```python
from build123d import *

# Parameters (mm, degrees)
SKETCH1_R           = 1.5
BOSS_EXTRUDE1_DEPTH = 0.5
SKETCH2_W           = 16.871696
SKETCH2_H           = 4.360926
SKETCH2_W_2         = 4.86899
SKETCH2_H_2         = 12.600052
CUT_EXTRUDE2_DEPTH  = 37.229212531
FILLET1_R           = 1
SKETCH3_R           = 1
SKETCH3_W           = 1.5
SKETCH3_H           = 4
SKETCH3_R_2         = 1.5
BOSS_EXTRUDE2_DEPTH = 2.05
FILLET2_R           = 1
FILLET4_R           = 0.75


# Some blends are built 0.0001 mm under size
with BuildPart() as part:
    # Sketch1 → Boss-Extrude1 (new body)
    with BuildSketch(Plane.XZ.offset(3.35)):
        with BuildLine():
            Line((-30.468062, -16.001619), (30.468062, -16.001619))
            ThreePointArc((30.468062, -16.001619), (31.904902979, -15.406459979), (32.500062, -13.969619))
            Line((32.500062, -13.969619), (32.500062, 13.969619))
            ThreePointArc((32.500062, 13.969619), (31.904902979, 15.406459979), (30.468062, 16.001619))
            Line((30.468062, 16.001619), (-30.468062, 16.001619))
            ThreePointArc((-30.468062, 16.001619), (-31.904902979, 15.406459979), (-32.500062, 13.969619))
            Line((-32.500062, 13.969619), (-32.500062, -13.969619))
            ThreePointArc((-32.500062, -13.969619), (-31.904902979, -15.406459979), (-30.468062, -16.001619))
        make_face()
        with Locations(Location((28.999942, -11.463655, 0), (0, 0, 270))):
            Circle(SKETCH1_R, mode=Mode.SUBTRACT)
        with Locations(Location((28.999942, 11.536299, 0), (0, 0, 270))):
            Circle(SKETCH1_R, mode=Mode.SUBTRACT)
        with Locations(Location((-29.000196, -11.463655, 0), (0, 0, 270))):
            Circle(SKETCH1_R, mode=Mode.SUBTRACT)
        with Locations(Location((-29.000196, 11.536299, 0), (0, 0, 270))):
            Circle(SKETCH1_R, mode=Mode.SUBTRACT)
    extrude(amount=-BOSS_EXTRUDE1_DEPTH)

    # Sketch2 → Cut-Extrude2 (cut, through all)
    with BuildSketch(Plane.XZ.offset(3.35)):
        with Locations((-4.81203, 13.821156)):
            Rectangle(SKETCH2_W, SKETCH2_H)
        Polygon((-20.66863, -8.001619), (10.02857, -8.001619), (10.02857, -16.001619), (-25.94464, -16.001619), (-25.94464, -11.279987), (-20.66863, -11.279987), align=None)
        with Locations((30.065567, 1.825117)):
            Rectangle(SKETCH2_W_2, SKETCH2_H_2)
    extrude(amount=-CUT_EXTRUDE2_DEPTH, mode=Mode.SUBTRACT)

    # Fillet1
    fillet1_edges = [part.edges().sort_by_distance(p)[0] for p in [
        (-13.247878, -3.1, 16.001619),
        (3.623818, -3.1, 16.001619),
        (-20.66863, -3.1, -11.279987),
        (10.02857, -3.1, -16.001619),
        (-25.94464, -3.1, -16.001619),
        (32.500062, -3.1, 8.125143),
        (32.500062, -3.1, -4.474909),
    ]]
    fillet(fillet1_edges, radius=FILLET1_R)

    # Sketch3 → Boss-Extrude2 (add)
    # profile 1 of 9: a face of its own
    with BuildSketch(Plane.XZ.offset(3.35)):
        with Locations(Location((-12.947878, 8.140693, 0), (0, 0, 270))):
            Circle(SKETCH3_R)
    # profile 2 of 9: a face of its own
    with BuildSketch(Plane.XZ.offset(3.35)):
        with Locations(Location((-18.447878, 15.001619, 0), (0, 0, 90))):
            Circle(SKETCH3_R)
    # profile 3 of 9: a face of its own
    with BuildSketch(Plane.XZ.offset(3.35)):
        with Locations(Location((5.356479, 14.268958, 0), (0, 0, 270))):
            Circle(SKETCH3_R)
    # profile 4 of 9: a face of its own
    with BuildSketch(Plane.XZ.offset(3.35)):
        Polygon((-20.46863, -8.001619), (9.02857, -8.001619), (9.02857, -6.501619), (4.02857, -6.501619), (4.02857, 8.498381), (7.52857, 8.498381), (7.52857, 9.998381), (-0.47143, 9.998381), (-0.47143, 8.498381), (2.52857, 8.498381), (2.52857, -6.501619), (-20.46863, -6.501619), align=None)
    # profile 5 of 9: a face of its own
    with BuildSketch(Plane.XZ.offset(3.35)):
        with Locations((15.204059, 14.001619)):
            Rectangle(SKETCH3_W, SKETCH3_H)
    # profile 6 of 9: a face of its own
    with BuildSketch(Plane.XZ.offset(3.35)):
        with BuildLine():
            Line((-32.500062, -3.797223), (-32.500062, -13.969619))
            ThreePointArc((-32.500062, -13.969619), (-31.904902979, -15.406459979), (-30.468062, -16.001619))
            Line((-30.468062, -16.001619), (-26.94464, -16.001619))
            ThreePointArc((-26.94464, -16.001619), (-26.237533219, -15.708725781), (-25.94464, -15.001619))
            Line((-25.94464, -15.001619), (-25.94464, -8.001619))
            Line((-25.94464, -8.001619), (-31.000062, -8.001619))
            Line((-31.000062, -8.001619), (-31.000062, -3.797223))
            Line((-31.000062, -3.797223), (-32.500062, -3.797223))
        make_face()
        with Locations(Location((-29.000196, -11.463655, 0), (0, 0, 270))):
            Circle(SKETCH3_R_2, mode=Mode.SUBTRACT)
    # profile 7 of 9: a face of its own
    with BuildSketch(Plane.XZ.offset(3.35)):
        with BuildLine():
            Line((32.500062, -5.474909), (31.000062, -5.474909))
            Line((31.000062, -5.474909), (31.000062, -9.001619))
            Line((31.000062, -9.001619), (25.569228, -9.001619))
            Line((25.569228, -9.001619), (25.569228, -16.001619))
            Line((25.569228, -16.001619), (30.468062, -16.001619))
            ThreePointArc((30.468062, -16.001619), (31.904902979, -15.406459979), (32.500062, -13.969619))
            Line((32.500062, -13.969619), (32.500062, -5.474909))
        make_face()
        with Locations(Location((28.999942, -11.463655, 0), (0, 0, 270))):
            Circle(SKETCH3_R_2, mode=Mode.SUBTRACT)
    # profile 8 of 9: a face of its own
    with BuildSketch(Plane.XZ.offset(3.35)):
        with BuildLine():
            Line((27.631072, 8.125143), (27.631072, 9.625143))
            Line((27.631072, 9.625143), (26.131072, 9.625143))
            Line((26.131072, 9.625143), (26.131072, 16.001619))
            Line((26.131072, 16.001619), (30.468062, 16.001619))
            ThreePointArc((30.468062, 16.001619), (31.904902979, 15.406459979), (32.500062, 13.969619))
            Line((32.500062, 13.969619), (32.500062, 9.125143))
            ThreePointArc((32.500062, 9.125143), (32.207168781, 8.418036219), (31.500062, 8.125143))
            Line((31.500062, 8.125143), (27.631072, 8.125143))
        make_face()
        with Locations(Location((28.999942, 11.536299, 0), (0, 0, 270))):
            Circle(SKETCH3_R_2, mode=Mode.SUBTRACT)
    # profile 9 of 9: a face of its own
    with BuildSketch(Plane.XZ.offset(3.35)):
        with BuildLine():
            Line((-32.500062, 8.102777), (-25.250062, 8.102777))
            Line((-25.250062, 8.102777), (-25.250062, 10.602777))
            Line((-25.250062, 10.602777), (-24.750062, 10.602777))
            Line((-24.750062, 10.602777), (-24.750062, 16.001619))
            Line((-24.750062, 16.001619), (-26.250062, 16.001619))
            Line((-26.250062, 16.001619), (-26.250062, 13.958671))
            Line((-26.250062, 13.958671), (-31.500062, 13.958671))
            ThreePointArc((-31.500062, 13.958671), (-32.207168781, 13.665777781), (-32.500062, 12.958671))
            Line((-32.500062, 12.958671), (-32.500062, 8.102777))
        make_face()
        with Locations(Location((-29.000196, 11.536299, 0), (0, 0, 270))):
            Circle(SKETCH3_R_2, mode=Mode.SUBTRACT)
    extrude(amount=-BOSS_EXTRUDE2_DEPTH)

    # Fillet2
    # the kernel refuses this fillet: 1 mm, written as the material it adds along each edge
    with BuildSketch(Plane(origin=(4.02857, -5.35, -6.501619), x_dir=(1, 0, 0), z_dir=(0, 1, 0))) as fillet2_piece_1_section:
        with BuildLine():
            CenterArc((FILLET2_R, -FILLET2_R), FILLET2_R, 90, 90)
            Line((0, -FILLET2_R), (0, 0))
            Line((0, 0), (FILLET2_R, 0))
        make_face()
    fillet2_piece_1 = extrude(amount=4.05, mode=Mode.PRIVATE)
    fillet2_piece_1 = split(fillet2_piece_1, bisect_by=Plane(origin=(4.02857, -3.35, -6.501619), z_dir=(0, 1, 0)), keep=Keep.TOP, mode=Mode.PRIVATE)
    add(fillet2_piece_1)
    with BuildSketch(Plane(origin=(2.52857, -5.35, -6.501619), x_dir=(0, 0, 1), z_dir=(0, 1, 0))) as fillet2_piece_2_section:
        with BuildLine():
            CenterArc((FILLET2_R, -FILLET2_R), FILLET2_R, 90, 90)
            Line((0, -FILLET2_R), (0, 0))
            Line((0, 0), (FILLET2_R, 0))
        make_face()
    fillet2_piece_2 = extrude(amount=4.05, mode=Mode.PRIVATE)
    fillet2_piece_2 = split(fillet2_piece_2, bisect_by=Plane(origin=(2.52857, -3.35, -6.501619), z_dir=(0, 1, 0)), keep=Keep.TOP, mode=Mode.PRIVATE)
    add(fillet2_piece_2)
    with BuildSketch(Plane(origin=(2.52857, -5.35, 8.498381), x_dir=(-1, 0, 0), z_dir=(0, 1, 0))) as fillet2_piece_3_section:
        with BuildLine():
            CenterArc((FILLET2_R, -FILLET2_R), FILLET2_R, 90, 90)
            Line((0, -FILLET2_R), (0, 0))
            Line((0, 0), (FILLET2_R, 0))
        make_face()
    fillet2_piece_3 = extrude(amount=4.05, mode=Mode.PRIVATE)
    fillet2_piece_3 = split(fillet2_piece_3, bisect_by=Plane(origin=(2.52857, -3.35, 8.498381), z_dir=(0, 1, 0)), keep=Keep.TOP, mode=Mode.PRIVATE)
    add(fillet2_piece_3)
    with BuildSketch(Plane(origin=(4.02857, -5.35, 8.498381), x_dir=(0, 0, -1), z_dir=(0, 1, 0))) as fillet2_piece_4_section:
        with BuildLine():
            CenterArc((FILLET2_R, -FILLET2_R), FILLET2_R, 90, 90)
            Line((0, -FILLET2_R), (0, 0))
            Line((0, 0), (FILLET2_R, 0))
        make_face()
    fillet2_piece_4 = extrude(amount=4.05, mode=Mode.PRIVATE)
    fillet2_piece_4 = split(fillet2_piece_4, bisect_by=Plane(origin=(4.02857, -3.35, 8.498381), z_dir=(0, 1, 0)), keep=Keep.TOP, mode=Mode.PRIVATE)
    add(fillet2_piece_4)
    with BuildSketch(Plane(origin=(-26.250062, -5.35, 13.958671), x_dir=(-1, 0, 0), z_dir=(0, 1, 0))) as fillet2_piece_5_section:
        with BuildLine():
            CenterArc((FILLET2_R, FILLET2_R), FILLET2_R, 180, 90)
            Line((0, FILLET2_R), (0, 0))
            Line((0, 0), (FILLET2_R, 0))
        make_face()
    fillet2_piece_5 = extrude(amount=4.05, mode=Mode.PRIVATE)
    fillet2_piece_5 = split(fillet2_piece_5, bisect_by=Plane(origin=(-26.250062, -3.35, 13.958671), z_dir=(0, 1, 0)), keep=Keep.TOP, mode=Mode.PRIVATE)
    add(fillet2_piece_5)
    # the kernel refuses this fillet: 1 mm, written as the material it takes off along each edge
    with BuildSketch(Plane(origin=(-25.94464, -2.85, -8.001619), x_dir=(0, 0, -1), z_dir=(0, 1, 0)), Plane(origin=(26.131072, -2.85, 16.001619), x_dir=(1, 0, 0), z_dir=(0, 1, 0)), Plane(origin=(26.131072, -2.85, 9.625143), x_dir=(0, 0, 1), z_dir=(0, 1, 0)), Plane(origin=(-25.250062, -2.85, 8.102777), x_dir=(-1, 0, 0), z_dir=(0, 1, 0))) as fillet2_2_piece_1:
        with BuildLine():
            CenterArc((FILLET2_R, FILLET2_R), FILLET2_R, 180, 90)
            Line((0, FILLET2_R), (0, 0))
            Line((0, 0), (FILLET2_R, 0))
        make_face()
    extrude(amount=4.05, mode=Mode.SUBTRACT)
    with BuildSketch(Plane(origin=(25.569228, -2.85, -16.001619), x_dir=(1, 0, 0), z_dir=(0, 1, 0)), Plane(origin=(25.569228, -2.85, -9.001619), x_dir=(0, 0, -1), z_dir=(0, 1, 0))) as fillet2_2_piece_2:
        with BuildLine():
            CenterArc((FILLET2_R, -FILLET2_R), FILLET2_R, 90, 90)
            Line((0, -FILLET2_R), (0, 0))
            Line((0, 0), (FILLET2_R, 0))
        make_face()
    extrude(amount=4.05, mode=Mode.SUBTRACT)
    with BuildSketch(Plane(origin=(-24.750062, -2.85, 10.602777), x_dir=(0, 0, 1), z_dir=(0, 1, 0))) as fillet2_2_piece_3:
        with BuildLine():
            CenterArc((0.866025404, -1), FILLET2_R, 90, 60)
            Line((0, -0.5), (0, 0))
            Line((0, 0), (0.866025404, 0))
        make_face()
    extrude(amount=3.715063509, mode=Mode.SUBTRACT)

    # Fillet4
    fillet4_edges = [part.edges().sort_by_distance(p)[0] for p in [
        (-31.000062, -2.075, -8.001619),
        (-20.46863, -2.075, -8.001619),
        (-20.46863, -2.075, -6.501619),
        (-0.47143, -2.075, 8.498381),
        (-0.47143, -2.075, 9.998381),
        (7.52857, -2.075, 9.998381),
        (7.52857, -2.075, 8.498381),
        (9.02857, -2.075, -8.001619),
        (9.02857, -2.075, -6.501619),
        (31.000062, -2.075, -9.001619),
        (31.000062, -2.075, -5.474909),
        (32.500062, -2.075, -5.474909),
        (27.631072, -2.075, 8.125143),
        (14.454059, -2.075, 12.001619),
        (15.954059, -2.075, 12.001619),
        (15.954059, -2.075, 16.001619),
        (14.454059, -2.075, 16.001619),
        (-32.500062, -2.075, 8.102777),
        (-24.750062, -2.075, 16.001619),
        (-26.250062, -2.075, 16.001619),
        (-31.000062, -2.075, -3.797223),
        (-32.500062, -2.075, -3.797223),
    ]]
    fillet(fillet4_edges, radius=FILLET4_R - 0.0001)  # a hair under: the kernel refuses the full size


solid = part.part
```
Geometry check sheet. Reference: the model listing, model coordinates, mm. A direction names the side the tool comes from. Coordinates: 2 decimals unless noted, no trailing zeros. Loops run counter-clockwise (first coordinate to the right, second up) from the corner with the lowest first, then second, coordinate; pieces in that order, holes last. Notation, with made-up numbers: (39, -38) - (49, -38) arc R28 cw to (49, -11) - close; hole circle Ø3 at (40.25, 7). An arc over 180 degrees is marked (long way). One line per item, written item: value. Start each with the question number.
(1) Mould release check, pull along X, two halves, no side actions. Record for faces 1 (the cylindrical face through (-27.735, -2.339, 10.73)), 2 (the flat face through (30, -1.3, 13)), 3 (the flat face through (4, -2, 9.998)): released by +X, released by -X, zero draft, split by the parting line, or undercut.
(2) Cross-section at C-C on y = -2.35. Count the separate pieces of the cut face and the enclosed holes in it, plus the area to 3 significant figures.
(3) Tool access check on faces 4 (the flat face through (-29, -2, -16.002)), 5 (the flat face through (14.454, -2, 14)), 6 (the flat face through (31, -2, -7)). Record the directions out of +Z, -Z, +X, -X, +Y, -Y that give a thin tool (end or side, any length) a straight path to the whole face; none if there is none.
(4) Cross-section at D-D on x = -8. Enter the section's corners in (y, z), plus the area to 3 significant figures.
(5) Cross-section at B-B on z = 1. Enter the section's corners in (x, y).
(6) Material ranges on line 1 (X direction, y = -3, z = -9.5); line 2 (X direction, y = -1.75, z = -13.5); line 3 (X direction, y = -2.6, z = -6), recorded low to high. Write a range as [from, to].
(7) Depth check by flat-ended pin: P1, Ø1.2, axis at y = -2, z = -1, coming from the +X side; P2, Ø0.5, axis at x = -29, y = -2.5, coming from the +Z side. Enter the tip coordinate at first touch or a pass-through.
(8) Cross-section at A-A on x = -15.5. Enter the section's corners in (y, z), plus the area to 3 significant figures.
Results below:
1. face 1: undercut
1. face 2: zero draft
1. face 3: undercut
2. separate pieces: 9
2. enclosed holes: 4
2. area: 268 mm2
3. face 4: -Z, +X, -X, +Y, -Y
3. face 5: +Z, -Z, +Y
3. face 6: +Y
4. outline: (-3.35, -8) - (-1.3, -8) - (-1.3, -6.5) - (-2.85, -6.5) - (-2.85, 11.64) - (-3.35, 11.64) - close
4. area: 12.1 mm2
5. outline: (-32.5, -3.35) - (27.63, -3.35) - (27.63, -2.85) - (4.03, -2.85) - (4.03, -1.3) - (2.53, -1.3) - (2.53, -2.85) - (-32.5, -2.85) - close
6. line 1: x = [-32.5, -20.67], [10.03, 32.5]
6. line 2: x = [-32.5, -25.94], [25.57, 32.5]
6. line 3: x = [-32.5, -31], [2.4, 4.16], [31.03, 32.47]
7. P1: stops at x = 4.03
7. P2: stops at z = 13.96
8. outline: (-3.35, -8) - (-1.3, -8) - (-1.3, -6.5) - (-2.85, -6.5) - (-2.85, 16) - (-3.35, 16) - close
8. area: 14.3 mm2
